Geometry check sheet. Reference: the model listing, model coordinates, mm. A direction names the side the tool comes from. Round coordinates to 2 decimals unless told otherwise and drop trailing zeros. Loops run counter-clockwise (first coordinate to the right, second up) from the corner with the lowest first, then second, coordinate; pieces in that order, holes last. Notation, with made-up numbers: (12.5, 50) -> (30.5, 50) arc R23 cw to (30.5, 61) -> close; hole circle Ø2 at (-12.5, -20). An arc over 180 degrees is marked (long way). Use one line per item in the form item = value.
from build123d import *

# Parameters (mm, degrees)
F0_R     = 10.5
F0_R_2   = 9
F1_DEPTH = 25
F2_DEPTH = 23
F3_R     = 2
F4_DEPTH = 25.001
F6_DEPTH = 15


with BuildPart() as f1:
    # F0 (on Top) → F1 (new body)
    with BuildSketch(Plane.XY):
        Circle(F0_R)
        Circle(F0_R_2, mode=Mode.SUBTRACT)
        Circle(F0_R_2)
    extrude(amount=F1_DEPTH)

    # F0 (on Top) → F2 (cut)
    with BuildSketch(Plane.XY):
        Circle(F0_R_2)
    extrude(amount=F2_DEPTH, mode=Mode.SUBTRACT)

    # F3 (on face) → F4 (cut, through all)
    with BuildSketch(Plane.XY.offset(25)):
        Circle(F3_R)
    extrude(amount=-F4_DEPTH, mode=Mode.SUBTRACT)

    # F5 (on face) → F6 (cut)
    with BuildSketch(Plane.XY):
        with BuildLine():
            Line((6.2500670258, 6.4758522352), (7.1391263091, 7.699537359))
            ThreePointArc((7.1391263091, 7.699537359), (6.1717451491, 8.4946784409), (5.1165838232, 9.1690004897))
            Line((5.1165838232, 9.1690004897), (4.2275245399, 7.945315366))
            ThreePointArc((4.2275245399, 7.945315366), (5.2900672706, 7.2811529494), (6.2500670258, 6.4758522352))
        make_face()
        with BuildLine():
            Line((8.8628208798, 1.5653772877), (10.3013490182, 2.0327834135))
            ThreePointArc((10.3013490182, 2.0327834135), (9.9860934211, 3.2446784409), (9.5288065322, 4.4104247042))
            Line((9.5288065322, 4.4104247042), (8.0902783938, 3.9430185785))
            ThreePointArc((8.0902783938, 3.9430185785), (8.5595086467, 2.7811529494), (8.8628208798, 1.5653772877))
        make_face()
        with BuildLine():
            ThreePointArc((1.25, 10.425329731), (0, 10.5), (-1.25, 10.425329731))
            Line((-1.25, 10.425329731), (-1.25, 8.912771735))
            ThreePointArc((-1.25, 8.912771735), (0, 9), (1.25, 8.912771735))
            Line((1.25, 8.912771735), (1.25, 10.425329731))
        make_face()
        with BuildLine():
            ThreePointArc((-5.1165838232, 9.1690004897), (-6.1717451491, 8.4946784409), (-7.1391263091, 7.699537359))
            Line((-7.1391263091, 7.699537359), (-6.2500670258, 6.4758522352))
            ThreePointArc((-6.2500670258, 6.4758522352), (-5.2900672706, 7.2811529494), (-4.2275245399, 7.945315366))
            Line((-4.2275245399, 7.945315366), (-5.1165838232, 9.1690004897))
        make_face()
        with BuildLine():
            ThreePointArc((-10.3013490182, -2.0327834135), (-9.9860934211, -3.2446784409), (-9.5288065322, -4.4104247042))
            Line((-9.5288065322, -4.4104247042), (-8.0902783938, -3.9430185785))
            ThreePointArc((-8.0902783938, -3.9430185785), (-8.5595086467, -2.7811529494), (-8.8628208798, -1.5653772877))
            Line((-8.8628208798, -1.5653772877), (-10.3013490182, -2.0327834135))
        make_face()
        with BuildLine():
            ThreePointArc((-7.1391263091, -7.699537359), (-6.1717451491, -8.4946784409), (-5.1165838232, -9.1690004897))
            Line((-5.1165838232, -9.1690004897), (-4.2275245399, -7.945315366))
            ThreePointArc((-4.2275245399, -7.945315366), (-5.2900672706, -7.2811529494), (-6.2500670258, -6.4758522352))
            Line((-6.2500670258, -6.4758522352), (-7.1391263091, -7.699537359))
        make_face()
        with BuildLine():
            Line((-1.25, -8.912771735), (-1.25, -10.425329731))
            ThreePointArc((-1.25, -10.425329731), (0, -10.5), (1.25, -10.425329731))
            Line((1.25, -10.425329731), (1.25, -8.912771735))
            ThreePointArc((1.25, -8.912771735), (0, -9), (-1.25, -8.912771735))
        make_face()
        with BuildLine():
            Line((4.2275245399, -7.945315366), (5.1165838232, -9.1690004897))
            ThreePointArc((5.1165838232, -9.1690004897), (6.1717451491, -8.4946784409), (7.1391263091, -7.699537359))
            Line((7.1391263091, -7.699537359), (6.2500670258, -6.4758522352))
            ThreePointArc((6.2500670258, -6.4758522352), (5.2900672706, -7.2811529494), (4.2275245399, -7.945315366))
        make_face()
        with BuildLine():
            ThreePointArc((-9.5288065322, 4.4104247042), (-9.9860934211, 3.2446784409), (-10.3013490182, 2.0327834135))
            Line((-10.3013490182, 2.0327834135), (-8.8628208798, 1.5653772877))
            ThreePointArc((-8.8628208798, 1.5653772877), (-8.5595086467, 2.7811529494), (-8.0902783938, 3.9430185785))
            Line((-8.0902783938, 3.9430185785), (-9.5288065322, 4.4104247042))
        make_face()
        Polygon((-0.7725424859, -1.0633135104), (-0.4774575141, -1.4694631307), (0, -1.3143277803), align=None)
        Polygon((0, -1.3143277803), (0.4774575141, -1.4694631307), (0.7725424859, -1.0633135104), align=None)
        with BuildLine():
            Line((8.0902783938, -3.9430185785), (9.5288065322, -4.4104247042))
            ThreePointArc((9.5288065322, -4.4104247042), (9.9860934211, -3.2446784409), (10.3013490182, -2.0327834135))
            Line((10.3013490182, -2.0327834135), (8.8628208798, -1.5653772877))
            ThreePointArc((8.8628208798, -1.5653772877), (8.5595086467, -2.7811529494), (8.0902783938, -3.9430185785))
        make_face()
    extrude(amount=F6_DEPTH, mode=Mode.SUBTRACT)


solid = f1.part
1. Gauge pin test, flat ends, axial feed: pin 1 (1.2 mm diameter, centred on y = 10, z = 9.5, fed in from -X); pin 2 (1.7 mm diameter, centred on y = -9.5, z = 11, fed in from -X); pin 3 (1.5 mm diameter, centred on y = -7.5, z = 13, fed in from +X). Record the tip position at first contact, or that the pin passes through.
Return value:
pin_1 = -4.68
pin_2 = -5.12
pin_3 = 8.04
2. Section check C-C (z = 2.5). Count the separate pieces of the cut face and the enclosed holes in it, then the cut area to 3 significant figures.
Return value:
separate_pieces = 10
enclosed_holes = 0
area = 54.3 mm2
3. Mould release check, pull along X, two halves, no side actions. Record for faces 6 (the flat face through (-8.799, 4.173, 7.395)), 7 (the flat face through (8, 6, 0)), 8 (the flat face through (9.59, -1.8, 7.4)): released by +X, released by -X, zero draft, split by the parting line, or undercut.
Return value:
face_6 = released by -X
face_7 = zero draft
face_8 = undercut
4. Tool access check on faces 1 (the flat face through (6.69, 7.08, 7.4)), 2 (the flat face through (-4.666, 8.549, 7.395)), 3 (the flat face through (-6, 8, 15)), 4 (the flat face through (-6.69, -7.08, 7.4)), 5 (the flat face through (-1.25, 10, 7)). Record the directions out of +Z, -Z, +X, -X, +Y, -Y that give a thin tool (end or side, any length) a straight path to the whole face; none if there is none.
Return value:
face_1 = -Z, +Y
face_2 = -Z, -X
face_3 = -Z
face_4 = -Z, -Y
face_5 = -Z, +Y, -Y
5. Section check A-A (y = 0). Record the boundary of the cut face in (x, z), then the cut area to 3 significant figures.
Return value:
outline = (-10.5, 0) -> (-9, 0) -> (-9, 23) -> (-2, 23) -> (-2, 25) -> (-10.5, 25) -> close; (2, 23) -> (9, 23) -> (9, 0) -> (10.5, 0) -> (10.5, 25) -> (2, 25) -> close
area = 103 mm2
6. Material ranges on line 1 along Y through (x, z) = (0, 23.6); line 2 along X through (y, z) = (0, 5.5); line 3 along Y through (x, z) = (-1.25, 20), recorded low to high.
Return value:
line_1 = -10.5 to -2, 2 to 10.5
line_2 = -10.5 to -9, 9 to 10.5
line_3 = -10.43 to -8.91, 8.91 to 10.43
7. Section check B-B (x = 0). Record the boundary of the cut face in (y, z).
Return value:
outline = (-10.5, 15) -> (-9, 15) -> (-9, 23) -> (-2, 23) -> (-2, 25) -> (-10.5, 25) -> close; (2, 23) -> (9, 23) -> (9, 15) -> (10.5, 15) -> (10.5, 25) -> (2, 25) -> close
